Can you work these out from the drawing? Everything is in mm from the part's minimum corner. Round coordinates to 2 decimals unless told otherwise and drop trailing zeros. Order: outer loops, then holes, each group sorted by start corner. A loop starts at its lowest first (then second) coordinate and runs counter-clockwise, first axis right, second up. Notation, with made-up numbers: (-31, 79) -> (2, 79) arc R14 cw to (2, 85) -> close; hole circle Ø11 at (8.25, -24). An arc over 180 degrees is marked (long way). One line per item, written item: value.
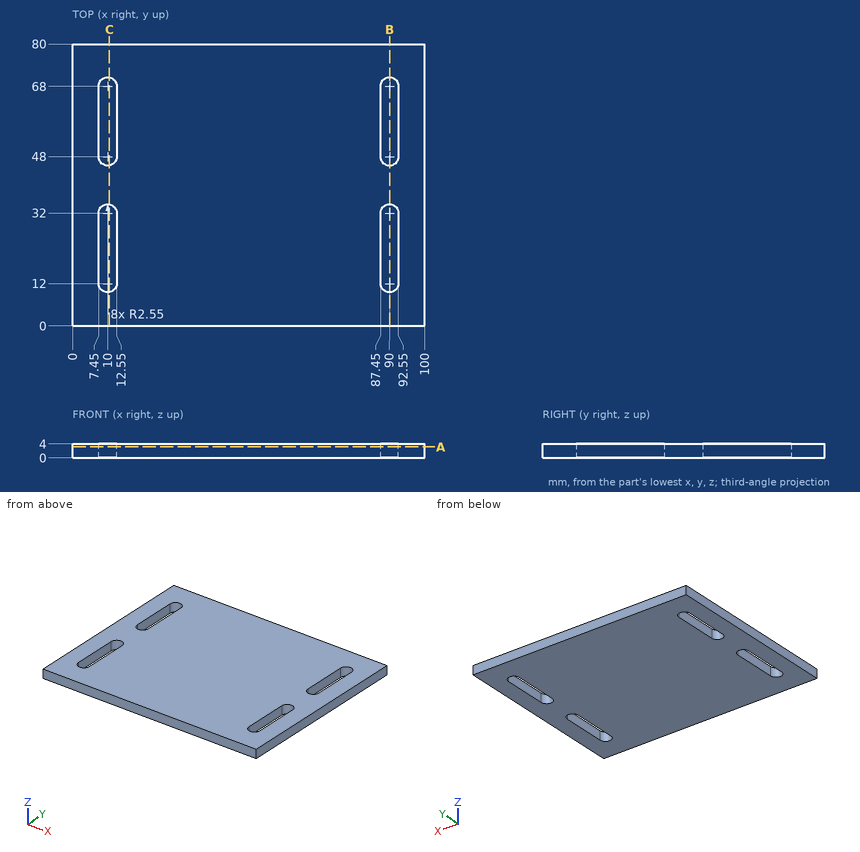
Q1. I want a section at C-C on x = 10.5. Write out the boundary of the cut face in (y, z), then the cut area to 3 significant figures.
Answers:
outline: (0, 0) -> (9.5, 0) -> (9.5, 4) -> (0, 4) -> close; (34.5, 0) -> (45.5, 0) -> (45.5, 4) -> (34.5, 4) -> close; (70.5, 0) -> (80, 0) -> (80, 4) -> (70.5, 4) -> close
area: 120 mm2
Q2. I need wall thicknesses on line 1 along X through (y, z) = (27, 2.4); line 2 along Y through (x, z) = (89, 0.7). Which ranges of each line are inside material? Lowest first, please.
Answers:
line 1: 0 to 7.45, 12.55 to 87.45, 92.55 to 100
line 2: 0 to 9.65, 34.35 to 45.65, 70.35 to 80
Q3. I want a section at A-A on z = 3.1. Write out the boundary of the cut face in (x, y), then the cut area to 3 significant figures.
Answers:
outline: (0, 0) -> (100, 0) -> (100, 80) -> (0, 80) -> close; hole (7.45, 12) arc R2.55 ccw to (12.55, 12) -> (12.55, 32) arc R2.55 ccw to (7.45, 32) -> close; hole (7.45, 48) arc R2.55 ccw to (12.55, 48) -> (12.55, 68) arc R2.55 ccw to (7.45, 68) -> close; hole (87.45, 12) arc R2.55 ccw to (92.55, 12) -> (92.55, 32) arc R2.55 ccw to (87.45, 32) -> close; hole (87.45, 48) arc R2.55 ccw to (92.55, 48) -> (92.55, 68) arc R2.55 ccw to (87.45, 68) -> close
area: 7,510 mm2
Q4. I want a section at B-B on x = 90. Write out the boundary of the cut face in (y, z).
Answers:
outline: (0, 0) -> (9.45, 0) -> (9.45, 4) -> (0, 4) -> close; (34.55, 0) -> (45.45, 0) -> (45.45, 4) -> (34.55, 4) -> close; (70.55, 0) -> (80, 0) -> (80, 4) -> (70.55, 4) -> close
Q5. For P1, Ø2, axis at y = 19, z = 1, coming from the -X side, with a flat end and sliding along its axis, tell me the tip position at first contact or that it passes through.
Answers:
P1: x = 0
